```python
from build123d import *

# Parameters (mm, degrees)
SKETCH_R           = 7.25
PAD_DEPTH          = 2
SKETCH001_R        = 3.75
SKETCH001_R_2      = 2.5
PAD001_DEPTH       = 4.2
SKETCH002_R        = 1.25
PAD002_DEPTH       = 15
PAD003_DEPTH       = 1.5
POLARPATTERN_COUNT = 4


with BuildPart() as part:
    # Sketch → Pad (new body)
    with BuildSketch(Plane.XY):
        Circle(SKETCH_R)
    extrude(amount=PAD_DEPTH)

    # Sketch001 (on Face3 of Pad) → Pad001 (join)
    with BuildSketch(Plane.XY.offset(2)):
        Circle(SKETCH001_R)
        Circle(SKETCH001_R_2, mode=Mode.SUBTRACT)
    extrude(amount=PAD001_DEPTH)

    # Sketch002 (on Face7 of Pad001) → Pad002 (join)
    with BuildSketch(Plane.XY.offset(2)):
        Circle(SKETCH002_R)
    extrude(amount=PAD002_DEPTH)

    # Sketch003 (on Face3 of Pad002) → Pad003 (join)
    with BuildSketch(Plane.XY.offset(2)):
        with BuildLine():
            Line((-1, 3.614208), (-1, 6.114208))
            Line((-1, 6.114208), (1, 6.114208))
            Line((1, 6.114208), (1, 3.614208))
            ThreePointArc((1, 3.614208), (0, 3.75), (-1, 3.614208))
        make_face()
    pad003 = extrude(amount=PAD003_DEPTH)

    # PolarPattern: Pad003 ×4 about axis
    polarpattern_axis = Axis((0, 0, 2), (0, 0, 1))
    for i in range(1, POLARPATTERN_COUNT):
        add(pad003.rotate(polarpattern_axis, i * 360 / POLARPATTERN_COUNT))


solid = part.part
```
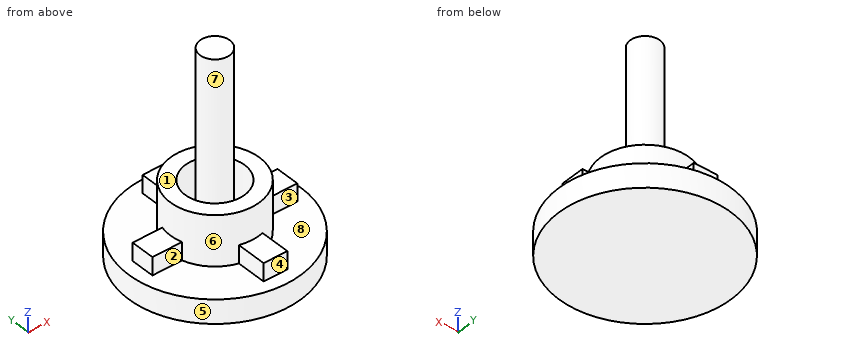
CAD build for the part. Positions are in the model's coordinates, mm. Face numbers are marked on the shaded views. A direction names the side the tool comes from. Coordinates: 2 decimals unless noted, no trailing zeros. Write each loop counter-clockwise with the first axis right and the second up, starting at its lowest first coordinate (ties: lowest second). Pieces come first, ordered by that corner, then holes. Notation, with made-up numbers: (-34, 62.25) -> (-4, 62.25) arc R12 cw to (-4, 80.25) -> close; hole circle Ø7 at (-18, 73.25). An arc over 180 degrees is marked (long way). Return JSON: item names as keys, results as strings. Group by question number.
Q1. Drill centre lines: line 1 (Y direction, x = 0, z = 4.5); line 2 (Y direction, x = 0, z = 3.45); line 3 (Z direction, x = 6, y = -2.25). Where is each one in solid material? Low to high.
Q2. Which spindle directions (+Z, -Z, +X, -X, +Y, -Y) get a long thin tool onto all of the face, cutting with end or side? Do the marked faces 1, 2, 3, 4 and 5. Say none if no direction does.
Q3. Cut at B-B, the plane x = 0. Give the cut face in (y, z), then the cut area to 3 significant figures.
Q4. Flat gauge pins, fed straight in: pin 1 (1.6 mm diameter, centred on x = -5, z = 3, fed in from +Y); pin 2 (6 mm diameter, centred on x = -3.5, y = -4, fed in from +Z); pin 3 (2 mm diameter, centred on x = -5.5, y = 0, fed in from +Z); pin 4 (3 mm diameter, centred on x = 3.5, z = 8, fed in from +Y). Where does each tip first touch, or does it go through?
Q5. Cut at A-A, the plane z = 2.5. Give the cut face in (x, y), then the cut area to 3 significant figures.
Q6. Pull direction X, two halves, no side cores. Call the marked faces 6, 7 and 8: released by +X, released by -X, zero draft, split by the parting line, or undercut.
Q7. Cut at D-D, the plane z = 7.25. Give the cut face in (x, y), then the cut area to 3 significant figures.
Returned:
{
 "1": {"line 1": "y = -3.75 to -2.5, -1.25 to 1.25, 2.5 to 3.75", "line 2": "y = -6.11 to -2.5, -1.25 to 1.25, 2.5 to 6.11", "line 3": "z = 0 to 2"},
 "2": {"face 1": "+Z", "face 2": "+Z, -X, -Y", "face 3": "+Z, +X, -Y", "face 4": "+Z, +X, -X, -Y", "face 5": "+Z, -Z"},
 "3": {"outline": "(-7.25, 0) -> (7.25, 0) -> (7.25, 2) -> (6.11, 2) -> (6.11, 3.5) -> (3.75, 3.5) -> (3.75, 6.2) -> (2.5, 6.2) -> (2.5, 2) -> (1.25, 2) -> (1.25, 17) -> (-1.25, 17) -> (-1.25, 2) -> (-2.5, 2) -> (-2.5, 6.2) -> (-3.75, 6.2) -> (-3.75, 3.5) -> (-6.11, 3.5) -> (-6.11, 2) -> (-7.25, 2) -> close", "area": "84.1 mm2"},
 "4": {"pin 1": "stops at y = 1", "pin 2": "stops at z = 6.2", "pin 3": "stops at z = 3.5", "pin 4": "passes through"},
 "5": {"outline": "(-6.11, -1) -> (-3.61, -1) arc R3.75 ccw to (-1, -3.61) -> (-1, -6.11) -> (1, -6.11) -> (1, -3.61) arc R3.75 ccw to (3.61, -1) -> (6.11, -1) -> (6.11, 1) -> (3.61, 1) arc R3.75 ccw to (1, 3.61) -> (1, 6.11) -> (-1, 6.11) -> (-1, 3.61) arc R3.75 ccw to (-3.61, 1) -> (-6.11, 1) -> close; circle Ø2.5 at (0, 0); hole circle Ø5 at (0, 0)", "area": "48.7 mm2"},
 "6": {"face 6": "split by the parting line", "face 7": "undercut", "face 8": "zero draft"},
 "7": {"outline": "circle Ø2.5 at (0, 0)", "area": "4.91 mm2"}
}
